Source: CAD feature listing. Evaluate the final solid. Frame: model axes, mm. A direction names the side the tool comes from. Coordinates: 2 decimals unless noted, no trailing zeros. Loops run counter-clockwise (first coordinate to the right, second up) from the corner with the lowest first, then second, coordinate; pieces in that order, holes last. Notation, with made-up numbers: (57.25, -32.5) -> (68.25, -32.5) arc R15 ccw to (68.25, -20.5) -> close; hole circle Ø9 at (-26.75, 71.25). An arc over 180 degrees is marked (long way). Answer as a JSON object with one key per item and string values. Group by question number.
from build123d import *

# Parameters (mm, degrees)
SKETCH1_R           = 1.016
SKETCH1_R_2         = 0.508
SKETCH1_R_3         = 0.9398
BOSS_EXTRUDE1_DEPTH = 0.8128
BOSS_EXTRUDE2_DEPTH = 2.794
SKETCH3_R           = 2.667
BOSS_EXTRUDE3_DEPTH = 2.54
FILLET1_R           = 2.54
BOSS_EXTRUDE4_START = -1.651
SKETCH4_R           = 1.397
SKETCH4_R_2         = 0.9398
SKETCH4_R_3         = 0.762
SKETCH4_R_4         = 0.508
BOSS_EXTRUDE4_DEPTH = 1.778
SKETCH5_W           = 5.08
SKETCH5_H           = 1.524
BOSS_EXTRUDE5_DEPTH = 1.651
CUT_EXTRUDE1_REACH  = 20.407
SKETCH7_W           = 2.8702
SKETCH7_H           = 1.143
BOSS_EXTRUDE6_DEPTH = 0.9398
SKETCH8_W           = 2.921
SKETCH8_H           = 2.794
BOSS_EXTRUDE7_DEPTH = 1.143
SKETCH9_W           = 1.397
SKETCH9_H           = 1.905
SKETCH9_W_2         = 1.905
SKETCH9_H_2         = 1.397
BOSS_EXTRUDE8_DEPTH = 1.651


with BuildPart() as part:
    # Sketch1 → Boss-Extrude1 (new, symmetric)
    with BuildSketch(Plane(origin=(0, 0, 0), x_dir=(1, 0, 0), z_dir=(0, 1, 0))):
        with BuildLine():
            Line((-10.541, 2.159), (-10.287, 2.159))
            ThreePointArc((-10.287, 2.159), (-9.927789755, 2.307789755), (-9.779, 2.667))
            Line((-9.779, 2.667), (-9.779, 4.826))
            ThreePointArc((-9.779, 4.826), (-9.035051224, 6.622051224), (-7.239, 7.366))
            Line((-7.239, 7.366), (-5.5118, 7.366))
            ThreePointArc((-5.5118, 7.366), (-5.062787194, 7.551987194), (-4.8768, 8.001))
            Line((-4.8768, 8.001), (-4.8768, 8.7376))
            ThreePointArc((-4.8768, 8.7376), (-4.504825612, 9.635625612), (-3.6068, 10.0076))
            Line((-3.6068, 10.0076), (3.6068, 10.0076))
            ThreePointArc((3.6068, 10.0076), (4.504825612, 9.635625612), (4.8768, 8.7376))
            Line((4.8768, 8.7376), (4.8768, 8.001))
            ThreePointArc((4.8768, 8.001), (5.062787194, 7.551987194), (5.5118, 7.366))
            Line((5.5118, 7.366), (7.239, 7.366))
            ThreePointArc((7.239, 7.366), (9.035051224, 6.622051224), (9.779, 4.826))
            Line((9.779, 4.826), (9.779, 2.667))
            ThreePointArc((9.779, 2.667), (9.927789755, 2.307789755), (10.287, 2.159))
            Line((10.287, 2.159), (10.414, 2.159))
            ThreePointArc((10.414, 2.159), (12.573, 0), (10.414, -2.159))
            Line((10.414, -2.159), (10.287, -2.159))
            ThreePointArc((10.287, -2.159), (9.927789755, -2.307789755), (9.779, -2.667))
            Line((9.779, -2.667), (9.779, -4.826))
            ThreePointArc((9.779, -4.826), (9.035051224, -6.622051224), (7.239, -7.366))
            Line((7.239, -7.366), (5.5118, -7.366))
            ThreePointArc((5.5118, -7.366), (5.062787194, -7.551987194), (4.8768, -8.001))
            Line((4.8768, -8.001), (4.8768, -8.7376))
            ThreePointArc((4.8768, -8.7376), (4.504825612, -9.635625612), (3.6068, -10.0076))
            Line((3.6068, -10.0076), (-3.6068, -10.0076))
            ThreePointArc((-3.6068, -10.0076), (-4.504825612, -9.635625612), (-4.8768, -8.7376))
            Line((-4.8768, -8.7376), (-4.8768, -8.001))
            ThreePointArc((-4.8768, -8.001), (-5.062787194, -7.551987194), (-5.5118, -7.366))
            Line((-5.5118, -7.366), (-7.239, -7.366))
            ThreePointArc((-7.239, -7.366), (-9.035051224, -6.622051224), (-9.779, -4.826))
            Line((-9.779, -4.826), (-9.779, -2.667))
            ThreePointArc((-9.779, -2.667), (-9.927789755, -2.307789755), (-10.287, -2.159))
            Line((-10.287, -2.159), (-10.541, -2.159))
            ThreePointArc((-10.541, -2.159), (-12.7, 0), (-10.541, 2.159))
        make_face()
        with Locations(Location((-10.541, 0, 0), (0, 0, 270))):
            Circle(SKETCH1_R, mode=Mode.SUBTRACT)
        with Locations(Location((10.414, 0, 0), (0, 0, 270))):
            Circle(SKETCH1_R, mode=Mode.SUBTRACT)
        with Locations(Location((0, 7.874, 0), (0, 0, 270))):
            Circle(SKETCH1_R_2, mode=Mode.SUBTRACT)
        with Locations(Location((0, -7.874, 0), (0, 0, 270))):
            Circle(SKETCH1_R_2, mode=Mode.SUBTRACT)
        with Locations(Location((-2.54, 7.874, 0), (0, 0, 270))):
            Circle(SKETCH1_R_3, mode=Mode.SUBTRACT)
        with Locations(Location((2.54, 7.874, 0), (0, 0, 270))):
            Circle(SKETCH1_R_3, mode=Mode.SUBTRACT)
        with Locations(Location((-2.54, -7.874, 0), (0, 0, 270))):
            Circle(SKETCH1_R_3, mode=Mode.SUBTRACT)
        with Locations(Location((2.54, -7.874, 0), (0, 0, 270))):
            Circle(SKETCH1_R_3, mode=Mode.SUBTRACT)
    extrude(amount=BOSS_EXTRUDE1_DEPTH, both=True)

    # Sketch2 → Boss-Extrude2 (add)
    with BuildSketch(Plane(origin=(0, 0.8128, 0), x_dir=(1, 0, 0), z_dir=(0, 1, 0))):
        with BuildLine():
            Line((-3.5941, 1.813922821), (-3.5941, -1.813922821))
            ThreePointArc((-3.5941, -1.813922821), (0, -4.0259), (3.5941, -1.813922821))
            Line((3.5941, -1.813922821), (3.5941, 1.813922821))
            ThreePointArc((3.5941, 1.813922821), (0, 4.0259), (-3.5941, 1.813922821))
        make_face()
    extrude(amount=BOSS_EXTRUDE2_DEPTH)

    # Sketch3 → Boss-Extrude3 (add)
    with BuildSketch(Plane(origin=(0, 3.6068, 0), x_dir=(1, 0, 0), z_dir=(0, 1, 0))):
        with Locations(Location((0, 0, 0), (0, 0, 270))):
            Circle(SKETCH3_R)
    extrude(amount=BOSS_EXTRUDE3_DEPTH)

    # Fillet1
    fillet1_edges = [part.edges().sort_by_distance(p)[0] for p in [
        (0, 6.1468, -2.667),
    ]]
    fillet(fillet1_edges, radius=FILLET1_R - 0.0001)  # a hair under: the kernel refuses the full size

    # Sketch4 → Boss-Extrude4 (add)
    # profile 1 of 6: a face of its own
    with BuildSketch(Plane(origin=(0, 0.8128, 0), x_dir=(1, 0, 0), z_dir=(0, 1, 0)).offset(BOSS_EXTRUDE4_START)):
        with Locations(Location((2.54, -7.874, 0), (0, 0, 270))):
            Circle(SKETCH4_R)
        with Locations(Location((2.54, -7.874, 0), (0, 0, 270))):
            Circle(SKETCH4_R_2, mode=Mode.SUBTRACT)
    # profile 2 of 6: a face of its own
    with BuildSketch(Plane(origin=(0, 0.8128, 0), x_dir=(1, 0, 0), z_dir=(0, 1, 0)).offset(BOSS_EXTRUDE4_START)):
        with Locations(Location((0, -7.874, 0), (0, 0, 270))):
            Circle(SKETCH4_R_3)
        with Locations(Location((0, -7.874, 0), (0, 0, 270))):
            Circle(SKETCH4_R_4, mode=Mode.SUBTRACT)
    # profile 3 of 6: a face of its own
    with BuildSketch(Plane(origin=(0, 0.8128, 0), x_dir=(1, 0, 0), z_dir=(0, 1, 0)).offset(BOSS_EXTRUDE4_START)):
        with Locations(Location((-2.54, -7.874, 0), (0, 0, 270))):
            Circle(SKETCH4_R)
        with Locations(Location((-2.54, -7.874, 0), (0, 0, 270))):
            Circle(SKETCH4_R_2, mode=Mode.SUBTRACT)
    # profile 4 of 6: a face of its own
    with BuildSketch(Plane(origin=(0, 0.8128, 0), x_dir=(1, 0, 0), z_dir=(0, 1, 0)).offset(BOSS_EXTRUDE4_START)):
        with Locations(Location((-2.54, 7.874, 0), (0, 0, 270))):
            Circle(SKETCH4_R)
        with Locations(Location((-2.54, 7.874, 0), (0, 0, 270))):
            Circle(SKETCH4_R_2, mode=Mode.SUBTRACT)
    # profile 5 of 6: a face of its own
    with BuildSketch(Plane(origin=(0, 0.8128, 0), x_dir=(1, 0, 0), z_dir=(0, 1, 0)).offset(BOSS_EXTRUDE4_START)):
        with Locations(Location((0, 7.874, 0), (0, 0, 270))):
            Circle(SKETCH4_R_3)
        with Locations(Location((0, 7.874, 0), (0, 0, 270))):
            Circle(SKETCH4_R_4, mode=Mode.SUBTRACT)
    # profile 6 of 6: a face of its own
    with BuildSketch(Plane(origin=(0, 0.8128, 0), x_dir=(1, 0, 0), z_dir=(0, 1, 0)).offset(BOSS_EXTRUDE4_START)):
        with Locations(Location((2.54, 7.874, 0), (0, 0, 270))):
            Circle(SKETCH4_R)
        with Locations(Location((2.54, 7.874, 0), (0, 0, 270))):
            Circle(SKETCH4_R_2, mode=Mode.SUBTRACT)
    extrude(amount=BOSS_EXTRUDE4_DEPTH)

    # Sketch5 → Boss-Extrude5 (add)
    with BuildSketch(Plane(origin=(0, 0.8128, 0), x_dir=(1, 0, 0), z_dir=(0, 1, 0))):
        with Locations((6.1341, -1.051922821)):
            Rectangle(SKETCH5_W, SKETCH5_H)
        with Locations((6.1341, 1.051922821)):
            Rectangle(SKETCH5_W, SKETCH5_H)
        with Locations((-6.1341, 1.051922821)):
            Rectangle(SKETCH5_W, SKETCH5_H)
        with Locations((-6.1341, -1.051922821)):
            Rectangle(SKETCH5_W, SKETCH5_H)
    extrude(amount=BOSS_EXTRUDE5_DEPTH)

    # Cut-Extrude1: up to this face of the body (flat: up to its plane)
    cut_extrude1_end = Plane(part.part.faces().sort_by_distance((-6.1341, 1.6383, -1.813922821))[0])
    # Sketch6 → Cut-Extrude1 (cut, up to the picked face)
    with BuildSketch(Plane.XY.offset(1.813922821), mode=Mode.PRIVATE) as cut_extrude1_sk1:
        Polygon((-8.6741, 1.5748), (-3.5941, 2.4638), (-8.6741, 2.4638), align=None)
    cut_extrude1_tool1 = split(extrude(cut_extrude1_sk1.sketch, amount=-CUT_EXTRUDE1_REACH, mode=Mode.PRIVATE), bisect_by=cut_extrude1_end, keep=Keep.BOTH, mode=Mode.PRIVATE)
    # Sketch6 → Cut-Extrude1 (cut, up to the picked face)
    with BuildSketch(Plane.XY.offset(1.813922821), mode=Mode.PRIVATE) as cut_extrude1_sk2:
        Polygon((8.6741, 2.4638), (8.6741, 1.5748), (3.5941, 2.4638), align=None)
    cut_extrude1_tool2 = split(extrude(cut_extrude1_sk2.sketch, amount=-CUT_EXTRUDE1_REACH, mode=Mode.PRIVATE), bisect_by=cut_extrude1_end, keep=Keep.BOTH, mode=Mode.PRIVATE)
    add(cut_extrude1_tool1.solids().sort_by(Axis((-6.980767, 2.167467, 1.813923), (0, 0, -1)))[0], mode=Mode.SUBTRACT)
    add(cut_extrude1_tool2.solids().sort_by(Axis((6.980767, 2.167467, 1.813923), (0, 0, -1)))[0], mode=Mode.SUBTRACT)

    # Sketch7 → Boss-Extrude6 (add)
    with BuildSketch(Plane.XZ.offset(0.8128)):
        with Locations((7.2009, 4.1275)):
            Rectangle(SKETCH7_W, SKETCH7_H)
        with Locations((7.2009, -1.5875)):
            Rectangle(SKETCH7_W, SKETCH7_H)
        with Locations((3.2131, 2.2225)):
            Rectangle(SKETCH7_W, SKETCH7_H)
        with Locations((3.2131, -3.4925)):
            Rectangle(SKETCH7_W, SKETCH7_H)
        with Locations((-6.3119, -4.0005)):
            Rectangle(SKETCH7_W, SKETCH7_H)
        with Locations((-2.1971, -2.0955)):
            Rectangle(SKETCH7_W, SKETCH7_H)
    extrude(amount=BOSS_EXTRUDE6_DEPTH)

    # Sketch8 → Boss-Extrude7 (add)
    with BuildSketch(Plane(origin=(0, -0.8128, 0), x_dir=(-1, 0, 0), z_dir=(0, -1, 0))):
        with Locations((4.0005, -2.667)):
            Rectangle(SKETCH8_W, SKETCH8_H)
    extrude(amount=BOSS_EXTRUDE7_DEPTH)

    # Sketch9 → Boss-Extrude8 (add)
    with BuildSketch(Plane.XZ.offset(0.8128)):
        with Locations((-1.4605, 1.4605)):
            Rectangle(SKETCH9_W, SKETCH9_H)
        with Locations((-0.6477, 5.5245)):
            Rectangle(SKETCH9_W_2, SKETCH9_H_2)
    extrude(amount=BOSS_EXTRUDE8_DEPTH)


solid = part.part
1. Section query B-B on y = 3.25. Return loops of the section in (x, z), then the cut area to 3 significant figures.
2. Ray query, L1, parallel to Z at x = -2.5, y = -0.5; L2, parallel to X at y = -1.25, z = 1.5; L3, parallel to Y at x = 7.25, z = 5.5. Return the intervals inside material, ascending.
3. Section query A-A on x = 8. Return loops of the section in (y, z).
4. Pin query (flat end, axial travel): pin 1 Ø1.8 at (x, y) = (-5.5, 2) entering from +Z; pin 2 Ø2 at (y, z) = (1, -3.5) entering from -X; pin 3 Ø1.5 at (x, z) = (-3, -6.5) entering from -Y; pin 4 Ø1 at (x, y) = (-2.5, -1) entering from +Z. Return the tip coordinate at first contact, or that it passes through.
5. Section query C-C on x = -3. State how many separate pieces and enclosed holes the cut face has, then the cut area to 3 significant figures.
6. Mould query, pull axis Z, two halves, no side actions, for faces 4 (the face through (0.1, 0.813, 4.3)), 5 (the face through (3, 0.94, -9)), 6 (the face through (4.51, 0.01, 9.63)). Classes: pulls with the +Z half, pulls with the -Z half, needs draft (parallel to the pull), parting line crosses it, or undercut.
7. Reachability of faces 1 (the face through (2.2, 0, -7)), 2 (the face through (-1, -2, 0.508)), 3 (the face through (-3, -0.838, -9)) from +Z, -Z, +X, -X, +Y, -Y: full face, straight path, thin tool, end or side. Return the list, or none.
Solved:
{
 "1": {"outline": "(-3.59, -1.81) arc R4.03 ccw to (3.59, -1.81) -> (3.59, 1.81) arc R4.03 ccw to (-3.59, 1.81) -> close", "area": "48.8 mm^2"},
 "2": {"L1": "-10.01 to -8.81, -6.94 to 6.94, 8.81 to 10.01", "L2": "-5.46 to -2.54, -2.16 to -0.76", "L3": "-0.81 to 0.81"},
 "3": {"outline": "(-1.75, -2.16) -> (-0.81, -2.16) -> (-0.81, -7.25) -> (0.81, -7.25) -> (0.81, -1.81) -> (1.69, -1.81) -> (1.69, -0.29) -> (0.81, -0.29) -> (0.81, 0.29) -> (1.69, 0.29) -> (1.69, 1.81) -> (0.81, 1.81) -> (0.81, 7.25) -> (-0.81, 7.25) -> (-0.81, 4.7) -> (-1.75, 4.7) -> (-1.75, 3.56) -> (-0.81, 3.56) -> (-0.81, -1.02) -> (-1.75, -1.02) -> close"},
 "4": {"pin 1": "z = 1.81", "pin 2": "x = -9.8", "pin 3": "y = -0.84", "pin 4": "z = 10.01"},
 "5": {"separate pieces": "3", "enclosed holes": "0", "area": "46.8 mm^2"},
 "6": {"face 4": "undercut", "face 5": "needs draft", "face 6": "pulls with the +Z half"},
 "7": {"face 1": "+Y, -Y", "face 2": "+X, -X, -Y", "face 3": "-Z, +X, -X, -Y"}
}
